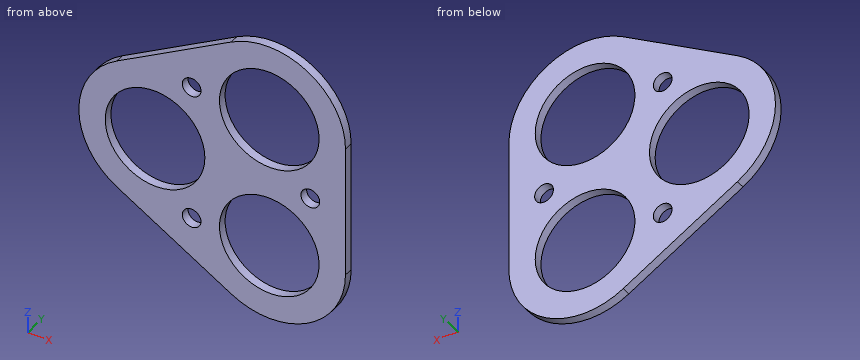
from build123d import *

# Parameters (mm, degrees)
SKETCH1_R           = 8.5
SKETCH1_R_2         = 1.6
SKETCH1_R_3         = 1.599999998
BOSS_EXTRUDE1_DEPTH = 1.5


with BuildPart() as part:
    # Sketch1 → Boss-Extrude1 (new body)
    with BuildSketch(Plane(origin=(0, 0, 0), x_dir=(1, 0, 0), z_dir=(0, 1, 0))):
        with BuildLine():
            Line((-15.804326324, -11.258330249), (3.681245261, -22.508330249))
            ThreePointArc((3.681245261, -22.508330249), (16.681245261, -22.508330249), (23.181245261, -11.25))
            Line((23.181245261, -11.25), (23.181245261, 11.25))
            ThreePointArc((23.181245261, 11.25), (16.681245261, 22.508330249), (3.681245261, 22.508330249))
            Line((3.681245261, 22.508330249), (-15.804326324, 11.258330249))
            ThreePointArc((-15.804326324, 11.258330249), (-22.304326324, 0), (-15.804326324, -11.258330249))
        make_face()
        with Locations((-9.304326324, 0)):
            Circle(SKETCH1_R, mode=Mode.SUBTRACT)
        with Locations((-3.06154027, 11.687177858)):
            Circle(SKETCH1_R_2, mode=Mode.SUBTRACT)
        with Locations((17.181245264, 0)):
            Circle(SKETCH1_R_3, mode=Mode.SUBTRACT)
        with Locations((10.181245261, -11.25)):
            Circle(SKETCH1_R, mode=Mode.SUBTRACT)
        with Locations((10.181245261, 11.25)):
            Circle(SKETCH1_R, mode=Mode.SUBTRACT)
        with Locations((-3.06154027, -11.687177373)):
            Circle(SKETCH1_R_2, mode=Mode.SUBTRACT)
    extrude(amount=BOSS_EXTRUDE1_DEPTH)


solid = part.part
Geometry check sheet. Reference: the model listing, model coordinates, mm. Coordinates: 2 decimals unless noted, no trailing zeros. Order: outer loops, then holes, each group sorted by start corner. A loop starts at its lowest first (then second) coordinate and runs counter-clockwise, first axis right, second up. Notation, with made-up numbers: M -20,41 L 1,41 A20 cw 1,52 Z; hole C 0.5,32 d1. An arc over 180 degrees is marked long. Use CSV: the item, a comma, the result in double quotes.
Item 1: Cross-section at C-C on z = 16. Record the cut outline in (x, y), then the cut area to 3 significant figures.
Returned:
outline,"M -7.59,0 L 3.13,0 L 3.13,1.5 L -7.59,1.5 Z; M 17.23,0 L 22.28,0 L 22.28,1.5 L 17.23,1.5 Z"
area,"23.7 mm2"
Item 2: Cross-section at A-A on z = 0. Record the cut outline in (x, y).
Returned:
outline,"M -22.3,0 L -17.8,0 L -17.8,1.5 L -22.3,1.5 Z; M -0.8,0 L 15.58,0 L 15.58,1.5 L -0.8,1.5 Z; M 18.78,0 L 23.18,0 L 23.18,1.5 L 18.78,1.5 Z"
Item 3: Thickness scan on line 1 along X through (y, z) = (0.3, 0); line 2 along X through (y, z) = (0.6, -6.5); line 3 along Z through (x, y) = (15.5, 0.55). Record the ranges inside material, lowest first.
Returned:
line 1,"x = -22.3 to -17.8, -0.8 to 15.58, 18.78 to 23.18"
line 2,"x = -20.56 to -14.78, -3.83 to 3.13, 17.23 to 23.18"
line 3,"z = -23.11 to -17.88, -4.62 to 4.62, 17.88 to 23.11"
Item 4: Cross-section at D-D on x = -15. Record the cut outline in (y, z).
Returned:
outline,"M 0,-11.72 L 1.5,-11.72 L 1.5,-6.31 L 0,-6.31 Z; M 0,6.31 L 1.5,6.31 L 1.5,11.72 L 0,11.72 Z"
Item 5: Cross-section at B-B on x = 10. Record the cut outline in (y, z).
Returned:
outline,"M 0,-24.25 L 1.5,-24.25 L 1.5,-19.75 L 0,-19.75 Z; M 0,-2.75 L 1.5,-2.75 L 1.5,2.75 L 0,2.75 Z; M 0,19.75 L 1.5,19.75 L 1.5,24.25 L 0,24.25 Z"
